Autodesk Inventor part; units mm, degrees
ref_plane "YZ Plane" through (0, 0, 0) normal (1, 0, 0) x (0, 1, 0)
ref_plane "XZ Plane" through (0, 0, 0) normal (0, 1, 0) x (-1, 0, 0)
ref_plane "XY Plane" through (0, 0, 0) normal (0, 0, 1) x (1, 0, 0)
ref_plane "Arbeitsebene1" through (0, 0, 0) normal (0, 0, 1) x (1, 0, 0)
sketch "Skizze1" plane through (0, 0, 0) normal (0, 0, 1) x (1, 0, 0)
  circle A0 centre (-42.2276, -19.25) radius 1.4
  circle A1 centre (-42.2276, -36.25) radius 1.4
  line L0 (-63.9, -22.9942) -> (-41.36, -22.9942)
  line L1 (-41.36, -32.5058) -> (-63.9, -32.5058)
  line L2 (-37.2276, -39.25) -> (-47.2276, -39.25)
  line L3 (-47.2276, -39.25) -> (-47.2276, -16.25)
  line L4 (-47.2276, -16.25) -> (-37.2276, -16.25)
  line L5 (-37.2276, -16.25) -> (-37.2276, -39.25)
  line L6 (-37.2276, -39.25) -> (-47.2276, -16.25) construction
  line L7 (-47.2276, -39.25) -> (-37.2276, -16.25) construction
  point P0 (0, 0)
  point P1 (-42.2276, -27.75)
  dimension "d0" = 10
  dimension "d1" = 3
  dimension "d2" = 3
extrude "Extrusion1" add sketch "Skizze1" along normal blind 3
fillet "Rundung1" radius 2 4 edges at (-37.2276, -16.25, 1.5) (-37.2276, -39.25, 1.5) (-47.2276, -39.25, 1.5) (-47.2276, -16.25, 1.5)
sketch "Skizze2" plane through (-37.2276, -37.25, 0) normal (1, 0, 0) x (0, 0, -1)
  line L0 (0, 13.5) -> (4.8526, 13.5)
  circle A0 centre (4.8526, 9.5) radius 7
  circle A1 centre (3.1016, 9.5) radius 4.5
  point P0 (0, 37.25)
  dimension "d6" = 9
extrude "Extrusion2" cut sketch "Skizze2" against normal through all contours A1
properties part number "20_Laserlauncher_Fixation"
Here's how the part is built. I have some questions about the finished solid (model axes, mm). Coordinates: 2 decimals unless noted, no trailing zeros. Order: outer loops, then holes, each group sorted by start corner. A loop starts at its lowest first (then second) coordinate and runs counter-clockwise, first axis right, second up. Notation, with made-up numbers: (3.5, -35) - (35.5, -35) arc R18 ccw to (35.5, -23) - close; hole circle Ø5 at (16, -2). An arc over 180 degrees is marked (long way). One line per question, with ' | ' between items. Start each with the question number.
1. Please list where these lines run through material, in increasing order: line 1 along Y through (x, z) = (-41.5, 2.55); line 2 along X through (y, z) = (-37.5, 2.5); line 3 along X through (y, z) = (-19, 2.7). Write a range as [from, to].
2. If we mould it in two halves opening along Y, with no side actions, what happens to faces 1 (the cylindrical face through (-46.626, -16.82, 1.521)), 2 (the flat face through (-42, -28, 3)), 3 (the cylindrical face through (-37.83, -38.68, 1.52)), 4 (the cylindrical face through (-40.934, -18.714, 1.479))? For each: released by +Y, released by -Y, zero draft, split by the parting line, or undercut.
3. If we section it at D-D (x = -42.75): Write out the boundary of the cut face in (y, z).
4. I'm going to push flat-ended pins straight in: pin 1 Ø3 at (x, y) = (-42.23, -36.25) entering from +Z; pin 2 Ø1.7 at (x, y) = (-42.23, -19.25) entering from +Z. Where does each tip first touch, or does it pass through?
5. If we section it at C-C (z = 1.15): Write out the boundary of the cut face in (x, y).
6. If we section it at B-B (z = 2.65): Write out the boundary of the cut face in (x, y), and give its area (3 significant figures).
7. If we section it at A-A (y = -36.25): Write out the boundary of the cut face in (x, z).
Model answer:
1) line 1: y = [-39.25, -37.45], [-35.05, -20.45], [-18.05, -16.25] | line 2: x = [-47.21, -42.86], [-41.6, -37.24] | line 3: x = [-47.23, -43.61], [-40.85, -37.23]
2) face 1: released by +Y | face 2: zero draft | face 3: released by -Y | face 4: undercut
3) outline: (-39.25, 0) - (-37.55, 0) - (-37.55, 3) - (-39.25, 3) - close; (-34.95, 0) - (-31.01, 0) arc R4.5 cw to (-24.49, 0) - (-20.55, 0) - (-20.55, 3) - (-34.95, 3) - close; (-17.95, 0) - (-16.25, 0) - (-16.25, 3) - (-17.95, 3) - close
4) pin 1: stops at z = 3 | pin 2: passes through
5) outline: (-47.23, -37.25) arc R2 ccw to (-45.23, -39.25) - (-39.23, -39.25) arc R2 ccw to (-37.23, -37.25) - (-37.23, -29.22) - (-47.23, -29.22) - close; (-47.23, -26.28) - (-37.23, -26.28) - (-37.23, -18.25) arc R2 ccw to (-39.23, -16.25) - (-45.23, -16.25) arc R2 ccw to (-47.23, -18.25) - close; hole circle Ø2.8 at (-42.23, -36.25); hole circle Ø2.8 at (-42.23, -19.25)
6) outline: (-47.23, -37.25) arc R2 ccw to (-45.23, -39.25) - (-39.23, -39.25) arc R2 ccw to (-37.23, -37.25) - (-37.23, -18.25) arc R2 ccw to (-39.23, -16.25) - (-45.23, -16.25) arc R2 ccw to (-47.23, -18.25) - close; hole circle Ø2.8 at (-42.23, -36.25); hole circle Ø2.8 at (-42.23, -19.25) | area: 214 mm²
7) outline: (-47.23, 0) - (-43.63, 0) - (-43.63, 3) - (-47.23, 3) - close; (-40.83, 0) - (-37.23, 0) - (-37.23, 3) - (-40.83, 3) - close
